from build123d import *

# Parameters (mm, degrees)
F0_W     = 127
F0_H     = 76.2
F0_R     = 6.35
F1_DEPTH = 50.8
F3_W     = 50.8
F3_H     = 25.4
F5_W     = 10.16
F5_H     = 10.16
F7_R     = 5.08


with BuildPart() as f1:
    # F0 (on Front) → F1 (new body)
    with BuildSketch(Plane.XZ):
        Rectangle(F0_W, F0_H)
        with Locations((-44.45, -19.05)):
            Circle(F0_R, mode=Mode.SUBTRACT)
        with Locations((44.45, -19.05)):
            Circle(F0_R, mode=Mode.SUBTRACT)
        with Locations((-44.45, 19.05)):
            Circle(F0_R, mode=Mode.SUBTRACT)
        with Locations((44.45, 19.05)):
            Circle(F0_R, mode=Mode.SUBTRACT)
    extrude(amount=F1_DEPTH)

    # F3 (on Right) → F4 (revolve)
    with BuildSketch(Plane.YZ):
        with Locations((25.4, -12.7)):
            Rectangle(F3_W, F3_H)
    revolve(axis=Axis((0, 25.4, 0), (0, 1, 0)))

    # F5 (on Right) → F6 (revolve, cut)
    with BuildSketch(Plane.YZ):
        with Locations((24.13, 20.32)):
            Rectangle(F5_W, F5_H)
    revolve(axis=Axis((0, 38.364865, 0), (0, 1, 0)), mode=Mode.SUBTRACT)

    # F7
    f7_edges = [f1.edges().sort_by_distance(p)[0] for p in [
        (63.5, 0, 0),
        (0, 0, 38.1),
        (0, 0, -38.1),
        (-63.5, 0, 0),
        (0, 19.05, 25.4),
        (0, 29.21, 25.4),
        (0, 50.8, 25.4),
    ]]
    fillet(f7_edges, radius=F7_R)


solid = f1.part
For this review, take the finished solid that the model builds, in its own axes (mm). A direction names the side the tool comes from. Round coordinates to 2 decimals unless told otherwise and drop trailing zeros. Order: outer loops, then holes, each group sorted by start corner. A loop starts at its lowest first (then second) coordinate and runs counter-clockwise, first axis right, second up. Notation, with made-up numbers: (70.5, 44) -> (106.5, 44) arc R18 cw to (106.5, 66) -> close; hole circle Ø10 at (-3, 10). An arc over 180 degrees is marked (long way). Write item = value, one per line. Start each with the question number.
1) Take a section at D-D on x = 0. State the section outline as (y, z) points, plus the area to 3 significant figures.
2) Tool access review of faces 1 (the face through (0.889, -1.449, -36.572)), 2 (the face through (15.15, 19.05, -2.92)), 3 (the face through (24.796, 40.085, 5.506)): name each direction out of +Z, -Z, +X, -X, +Y, -Y from which nothing blocks a thin tool from reaching the whole face with its end or side.
3) Take a section at B-B on y = -24. State the section outline as (x, z) points.
4) To check wall thickness, follow line 1 (X direction, y = -13, z = 18.5); line 2 (Z direction, x = 44, y = -13); line 3 (Y direction, x = -19, z = 3). State the ranges of each line that lie inside material, in increasing order. Write a range as from..to.
5) Take a section at C-C on z = -30.5. State the section outline as (x, y) points.
6) Insertion check: pin 1 (2 mm diameter, centred on y = 19.5, z = -7.5, fed in from +X); pin 2 (20.5 mm diameter, centred on x = -44.45, z = 19.05, fed in from -Y); pin 3 (3 mm diameter, centred on x = 27.5, y = 12, fed in from +Z); pin 4 (10 mm diameter, centred on x = -35, z = -10.5, fed in from +Y). Each pin has a flat end and moves straight along its axis. Give the tip position at first contact, or say it passes through.
7) Take a section at A-A on x = 44.45. State the section outline as (y, z) points.
8) The part is to be moulded in two halves that separate along Z. For faces 4 (the face through (-1, -50.8, 1)), 5 (the face through (-38.584, -25.044, -21.482)), 6 (the face through (-1, -28, -38.1)), say which applies: +Z half, -Z half, draft (parallel to the pull), parting line (faces both ways), or undercut.
Verdict:
q1.outline = (-50.8, -38.1) -> (-5.08, -38.1) arc R5.08 ccw to (0, -33.02) -> (0, -25.4) -> (13.97, -25.4) arc R5.08 ccw to (19.05, -20.32) -> (19.05, -15.24) -> (29.21, -15.24) -> (29.21, -20.32) arc R5.08 ccw to (34.29, -25.4) -> (45.72, -25.4) arc R5.08 ccw to (50.8, -20.32) -> (50.8, 20.32) arc R5.08 ccw to (45.72, 25.4) -> (34.29, 25.4) arc R5.08 ccw to (29.21, 20.32) -> (29.21, 15.24) -> (19.05, 15.24) -> (19.05, 20.32) arc R5.08 ccw to (13.97, 25.4) -> (0, 25.4) -> (0, 33.02) arc R5.08 ccw to (-5.08, 38.1) -> (-50.8, 38.1) -> close
q1.area = 6,200 mm2
q2.face_1 = -Z, +X, -X, +Y
q2.face_2 = none
q2.face_3 = +Y
q3.outline = (-63.5, -38.1) -> (63.5, -38.1) -> (63.5, 38.1) -> (-63.5, 38.1) -> close; hole circle Ø12.7 at (-44.45, -19.05); hole circle Ø12.7 at (-44.45, 19.05); hole circle Ø12.7 at (44.45, -19.05); hole circle Ø12.7 at (44.45, 19.05)
q4.line_1 = -63.5..-50.78, -38.12..38.12, 50.78..63.5
q4.line_2 = -38.1..-25.38, -12.72..12.72, 25.38..38.1
q4.line_3 = -50.8..19.05, 29.21..50.8
q5.outline = (-63.5, -50.8) -> (63.5, -50.8) -> (63.5, -5.08) arc R5.08 ccw to (58.42, 0) -> (-58.42, 0) arc R5.08 ccw to (-63.5, -5.08) -> close
q6.pin_1 = 21.37
q6.pin_2 = -50.8
q6.pin_3 = through
q6.pin_4 = 0
q7.outline = (-50.8, -38.1) -> (-5.08, -38.1) arc R5.08 ccw to (0, -33.02) -> (0, -25.4) -> (-50.8, -25.4) -> close; (-50.8, -12.7) -> (0, -12.7) -> (0, 12.7) -> (-50.8, 12.7) -> close; (-50.8, 25.4) -> (0, 25.4) -> (0, 33.02) arc R5.08 ccw to (-5.08, 38.1) -> (-50.8, 38.1) -> close
q8.face_4 = draft
q8.face_5 = undercut
q8.face_6 = -Z half
